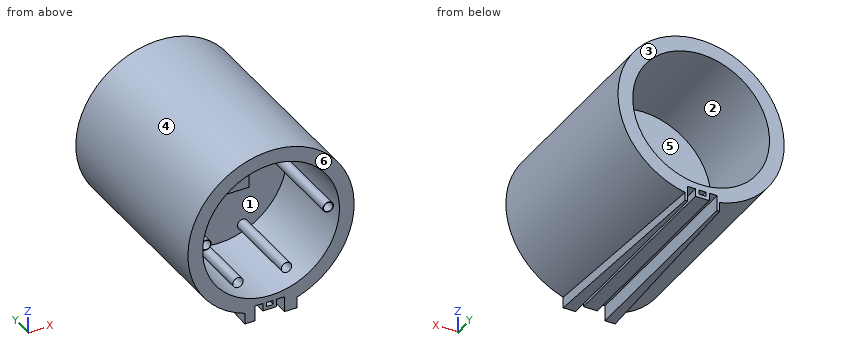
from build123d import *

# Parameters (mm, degrees)
SKETCH1_R           = 48
BOSS_EXTRUDE1_DEPTH = 115
SKETCH2_R           = 39.5
CUT_EXTRUDE3_DEPTH  = 115
SKETCH9_W           = 4.5
SKETCH9_H           = 9
CUT_EXTRUDE5_DEPTH  = 115
SKETCH14_W          = 4
SKETCH14_H          = 2.5
CUT_EXTRUDE8_DEPTH  = 115
SKETCH16_W          = 8
SKETCH16_H          = 4.5
CUT_EXTRUDE9_DEPTH  = 115
SKETCH19_R          = 41
BOSS_EXTRUDE2_DEPTH = 1
SKETCH21_R          = 3
BOSS_EXTRUDE3_DEPTH = 50
SHELL1_T            = -0.3
SKETCH24_R          = 3
BOSS_EXTRUDE4_DEPTH = 35
SHELL2_START        = 19
SHELL2_OUTLINE_R    = 2.7
SHELL2_DEPTH        = 35
SKETCH25_R          = 3
BOSS_EXTRUDE5_DEPTH = 45
SHELL5_T            = -0.03
SKETCH26_W          = 30
SKETCH26_H          = 15
BOSS_EXTRUDE6_DEPTH = 5


# Read off the part's stored shape, not the designer's step: Shell2
with BuildPart() as part:
    # Sketch1 → Boss-Extrude1 (new body)
    with BuildSketch(Plane(origin=(0, 0, 0), x_dir=(1, 0, 0), z_dir=(0, 1, 0))):
        with Locations(Location((0, 0, 0), (0, 0, 270))):
            Circle(SKETCH1_R)
    extrude(amount=BOSS_EXTRUDE1_DEPTH)

    # Sketch7 → Loft2 section 0
    with BuildSketch(Plane.XZ):
        with BuildLine():
            Line((-15.1377027, -38.271634302), (14.891561193, -38.271634302))
            Line((14.891561193, -38.271634302), (14.891561193, -51.96970786))
            Line((14.891561193, -51.96970786), (-15.1377027, -51.96970786))
            Line((-15.1377027, -51.96970786), (-15.1377027, -38.271634302))
        make_face()
    # Sketch6 → Loft2 section 1
    with BuildSketch(Plane(origin=(0, 115, 0), x_dir=(1, 0, 0), z_dir=(0, 1, 0))):
        with BuildLine():
            Line((-10.741203576, 39.96970786), (9.258796424, 39.96970786))
            Line((9.258796424, 39.96970786), (9.258796424, 51.96970786))
            Line((9.258796424, 51.96970786), (-10.741203576, 51.96970786))
            Line((-10.741203576, 51.96970786), (-10.741203576, 39.96970786))
        make_face()
    loft()

    # Sketch2 → Cut-Extrude3 (cut)
    with BuildSketch(Plane(origin=(0, 115, 0), x_dir=(1, 0, 0), z_dir=(0, 1, 0))):
        with Locations(Location((0, 0, 0), (0, 0, 270))):
            Circle(SKETCH2_R)
    extrude(amount=-CUT_EXTRUDE3_DEPTH, mode=Mode.SUBTRACT)

    # Sketch9 → Cut-Extrude5 (cut)
    with BuildSketch(Plane(origin=(0, 115, 0), x_dir=(1, 0, 0), z_dir=(0, 1, 0))):
        with Locations((-6.991203576, 47.46970786)):
            Rectangle(SKETCH9_W, SKETCH9_H)
        with Locations((5.508796424, 47.46970786)):
            Rectangle(SKETCH9_W, SKETCH9_H)
    extrude(amount=-CUT_EXTRUDE5_DEPTH, mode=Mode.SUBTRACT)

    # Sketch14 → Cut-Extrude8 (cut)
    with BuildSketch(Plane(origin=(0, 115, 0), x_dir=(1, 0, 0), z_dir=(0, 1, 0))):
        with Locations((-0.741203576, 44.290749204)):
            Rectangle(SKETCH14_W, SKETCH14_H)
    extrude(amount=-CUT_EXTRUDE8_DEPTH, mode=Mode.SUBTRACT)

    # Sketch16 → Cut-Extrude9 (cut)
    with BuildSketch(Plane(origin=(0, 115, 0), x_dir=(1, 0, 0), z_dir=(0, 1, 0))):
        with Locations((-0.741203576, 49.71970786)):
            Rectangle(SKETCH16_W, SKETCH16_H)
    extrude(amount=-CUT_EXTRUDE9_DEPTH, mode=Mode.SUBTRACT)

    # Sketch19 → Boss-Extrude2 (add)
    with BuildSketch(Plane(origin=(0, 54, 0), x_dir=(1, 0, 0), z_dir=(0, 1, 0))):
        Circle(SKETCH19_R)
    extrude(amount=BOSS_EXTRUDE2_DEPTH)

    # Sketch21 → Boss-Extrude3 (add)
    with BuildSketch(Plane.XZ.offset(-54)):
        with Locations(Location((-35.3, 0, 0), (0, 0, 90))):
            Circle(SKETCH21_R)
        with Locations(Location((35.3, 0, 0), (0, 0, 90))):
            Circle(SKETCH21_R)
    extrude(amount=BOSS_EXTRUDE3_DEPTH)

    # Shell1
    shell1_openings = [part.faces().sort_by_distance(p)[0] for p in [
        (-35.3, 4, 0),
        (35.3, 4, 0),
    ]]
    offset(amount=SHELL1_T, openings=shell1_openings, kind=Kind.INTERSECTION)

    # Sketch24 → Boss-Extrude4 (add)
    with BuildSketch(Plane.XZ.offset(-54)):
        with Locations(Location((7.5, 30, 0), (0, 0, 90))):
            Circle(SKETCH24_R)
        with Locations(Location((-7.5, 30, 0), (0, 0, 90))):
            Circle(SKETCH24_R)
    extrude(amount=BOSS_EXTRUDE4_DEPTH)

    # Shell2 outline → Shell2 (cut)
    with BuildSketch(Plane(origin=(0, 0, 0), x_dir=(1, 0, 0), z_dir=(0, 1, 0)).offset(SHELL2_START)):
        with Locations((-7.5, -30)):
            Circle(SHELL2_OUTLINE_R)
        with Locations((7.5, -30)):
            Circle(SHELL2_OUTLINE_R)
    extrude(amount=SHELL2_DEPTH, mode=Mode.SUBTRACT)

    # Sketch25 → Boss-Extrude5 (add)
    with BuildSketch(Plane.XZ.offset(-54)):
        with Locations(Location((14, -32.5, 0), (0, 0, 90))):
            Circle(SKETCH25_R)
        with Locations(Location((-14, -32.5, 0), (0, 0, 90))):
            Circle(SKETCH25_R)
    extrude(amount=BOSS_EXTRUDE5_DEPTH)

    # Shell5
    shell5_openings = [part.faces().sort_by_distance(p)[0] for p in [
        (-14, 9, -32.5),
        (14, 9, -32.5),
    ]]
    offset(amount=SHELL5_T, openings=shell5_openings, kind=Kind.INTERSECTION)

    # Sketch26 → Boss-Extrude6 (add)
    with BuildSketch(Plane.XZ.offset(-54)):
        Rectangle(SKETCH26_W, SKETCH26_H)
    extrude(amount=BOSS_EXTRUDE6_DEPTH)


solid = part.part
Input: part model. Units: mm. Frame: model coordinates. Face numbers are marked on the shaded views. A direction names the side the tool comes from. Give positions to 0.01 mm unless a question says otherwise; leave off trailing zeros. Loops run counter-clockwise (first coordinate to the right, second up) from the corner with the lowest first, then second, coordinate; pieces in that order, holes last. Notation, with made-up numbers: M 16,39.25 L 56,39.25 A28 ccw 56,61.25 Z; hole C 89.5,58 d11. An arc over 180 degrees is marked long. Use one line per item in the form item = value.
1. Section query D-D, the plane z = 42. Return the cut outline in (x, y), and give its area (3 significant figures).
Numbers:
outline = M -23.24,0 L 23.24,0 L 23.24,115 L -23.24,115 Z; M -22.67,0.27 L 22.67,0.27 L 22.67,114.73 L -22.67,114.73 Z; hole M -23.18,0.03 L 23.18,0.03 L 23.18,114.97 L -23.18,114.97 Z; hole M -22.61,0.3 L 22.61,0.3 L 22.61,114.7 L -22.61,114.7 Z
area = 34.2 mm²
2. Pull-direction query (Z, two-part tool) for the marked faces 4, 5 and 6; classes: released by +Z, released by -Z, zero draft, split by the parting line, or undercut.
Numbers:
face_4 = split by the parting line
face_5 = undercut
face_6 = zero draft
3. Reachability of the marked faces 1, 2 and 3 from +Z, -Z, +X, -X, +Y, -Y: full face, straight path, thin tool, end or side. Return the list, or none.
Numbers:
face_1 = -Y
face_2 = +Y
face_3 = +Z, -Z, +X, -X, +Y
4. First-contact query: pin 1 (3 mm diameter, centred on y = 14, z = 11.5, fed in from +X); pin 2 (6 mm diameter, centred on x = 25, y = 84.5, fed in from -Z); pin 3 (3 mm diameter, centred on x = -1.5, y = 60.5, fed in from +Z). Flat tips, straight axial feed; report the tip coordinate or a pass-through.
Numbers:
pin_1 = 46.95
pin_2 = -42.66
pin_3 = 48
5. Section query A-A, the plane z = 0. Count the separate pieces of the cut face and the enclosed holes in it, and give its area (3 significant figures).
Numbers:
separate_pieces = 2
enclosed_holes = 2
area = 200 mm²
